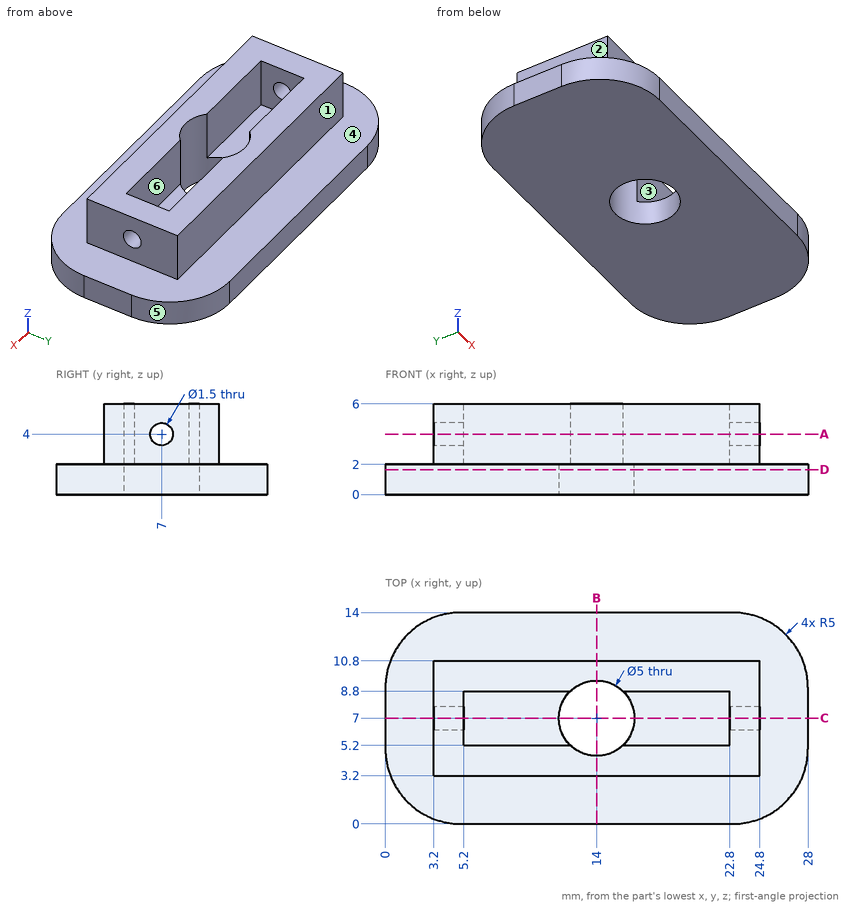
Study the drawing (mm; zero at the part's minimum x, y, z) and answer. A direction names the side the tool comes from. Round coordinates to 2 decimals unless told otherwise and drop trailing zeros. Write each loop counter-clockwise with the first axis right and the second up, starting at its lowest first coordinate (ties: lowest second). Pieces come first, ordered by that corner, then holes. Notation, with made-up numbers: (-5, 42.25) - (33, 42.25) arc R11 ccw to (33, 63.25) - close; hole circle Ø8 at (-8.5, 44.5). An arc over 180 degrees is marked (long way). Use a Markdown table: item, result. Add a question column.
1. Consider line 1 (Z direction, x = 3.85, y = 7); line 2 (Y direction, x = 14, z = 4.35); line 3 (X direction, y = 8.25, z = 2.6). Determine where each line is inside the solid, lowest interval first.
2. Flat-ended cylindrical pins translate along their axes: P1, Ø1.8, axis at x = 9, y = 7.5, coming from the +Z side; P2, Ø1.1, axis at y = 7.5, z = 4.5, coming from the +X side; P3, Ø1.2, axis at x = 19.5, z = 4, coming from the -Y side; P4, Ø0.9, axis at y = 7, z = 4, coming from the -X side. Find the tip coordinate at first contact, or state that the pin passes through.
3. A tool of negligible diameter and unlimited length cuts with its end or side. For the marked faces 1, 2 and 3, from which of +Z, -Z, +X, -X, +Y, -Y can it reach the whole face along a straight path? Write none if from no direction.
4. The part is cut by section C-C (y = 7). Write down the section's boundary in (x, z).
5. The part is cut by section D-D (z = 1.65). Write down the section's boundary in (x, y).
6. The part is cut by section B-B (x = 14). Write down the section's boundary in (y, z).
7. The part is cut by section A-A (z = 4). Write down the section's boundary in (x, y), and give its area (3 significant figures).
8. For a pull along Y with two mould halves and no side action, classify the marked faces 4, 5 and 6 as +Y half, -Y half, draft (parallel to the pull), parting line (faces both ways), or undercut.
Reported:
| question | item | result |
|---|---|---|
| 1 | line 1 | 0 to 3.25, 4.75 to 6 |
| 1 | line 2 | 3.2 to 4.5, 9.5 to 10.8 |
| 1 | line 3 | 3.2 to 5.2, 22.8 to 24.8 |
| 2 | P1 | z = 2 |
| 2 | P2 | x = 24.8 |
| 2 | P3 | y = 3.2 |
| 2 | P4 | through |
| 3 | face 1 | +Z, +X, -X, +Y |
| 3 | face 2 | +Z, -X, +Y, -Y |
| 3 | face 3 | +Z |
| 4 | outline | (0, 0) - (11.5, 0) - (11.5, 2) - (5.2, 2) - (5.2, 3.25) - (3.2, 3.25) - (3.2, 2) - (0, 2) - close; (3.2, 4.75) - (5.2, 4.75) - (5.2, 6) - (3.2, 6) - close; (16.5, 0) - (28, 0) - (28, 2) - (24.8, 2) - (24.8, 3.25) - (22.8, 3.25) - (22.8, 2) - (16.5, 2) - close; (22.8, 4.75) - (24.8, 4.75) - (24.8, 6) - (22.8, 6) - close |
| 5 | outline | (0, 5) arc R5 ccw to (5, 0) - (23, 0) arc R5 ccw to (28, 5) - (28, 9) arc R5 ccw to (23, 14) - (5, 14) arc R5 ccw to (0, 9) - close; hole circle Ø5 at (14, 7) |
| 6 | outline | (0, 0) - (4.5, 0) - (4.5, 6) - (3.2, 6) - (3.2, 2) - (0, 2) - close; (9.5, 0) - (14, 0) - (14, 2) - (10.8, 2) - (10.8, 6) - (9.5, 6) - close |
| 7 | outline | (3.2, 3.2) - (24.8, 3.2) - (24.8, 6.25) - (22.8, 6.25) - (22.8, 5.2) - (15.73, 5.2) arc R2.5 cw to (12.27, 5.2) - (5.2, 5.2) - (5.2, 6.25) - (3.2, 6.25) - close; (3.2, 7.75) - (5.2, 7.75) - (5.2, 8.8) - (12.27, 8.8) arc R2.5 cw to (15.73, 8.8) - (22.8, 8.8) - (22.8, 7.75) - (24.8, 7.75) - (24.8, 10.8) - (3.2, 10.8) - close |
| 7 | area | 91.5 mm^2 |
| 8 | face 4 | draft |
| 8 | face 5 | +Y half |
| 8 | face 6 | undercut |
